CAD build for the part. Positions are in the model's coordinates, mm. A direction names the side the tool comes from. Coordinates: 2 decimals unless noted, no trailing zeros. Write each loop counter-clockwise with the first axis right and the second up, starting at its lowest first coordinate (ties: lowest second). Pieces come first, ordered by that corner, then holes. Notation, with made-up numbers: M 35,42.5 L 70,42.5 A38 ccw 70,80.5 Z; hole C 80.5,-7.5 d7. An arc over 180 degrees is marked long. Answer as CSV lines item,"result". Start each with the question number.
Autodesk Inventor part; units mm, degrees
ref_plane "YZ Plane" through (0, 0, 0) normal (1, 0, 0) x (0, 1, 0)
ref_plane "XZ Plane" through (0, 0, 0) normal (0, 1, 0) x (-1, 0, 0)
ref_plane "XY Plane" through (0, 0, 0) normal (0, 0, 1) x (1, 0, 0)
sketch "Boceto1" plane through (0, 0, 0) normal (0, 0, 1) x (1, 0, 0)
  line L0 (98.53, 89.5715) -> (-98.53, 89.5715)
  line L1 (-98.53, -89.5715) -> (98.53, 89.5715) construction
  line L2 (98.53, -89.5715) -> (-98.53, 89.5715) construction
  line L3 (3.26, -89.5715) -> (3.26, -39.0815)
  line L4 (3.26, -39.0815) -> (98.53, -39.0815)
  line L5 (98.53, 89.5715) -> (98.53, -39.0815)
  circle A0 centre (65.96, 66.7715) radius 4.5
  circle A1 centre (65.96, -18.7285) radius 4.5
  circle A2 centre (-80.61, 72.0615) radius 4.5
  circle A3 centre (-4.48, 76.5415) radius 4.5
  circle A4 centre (-80.61, -22.7985) radius 4.5
  circle A5 centre (-4.48, -40.0285) radius 4.5
  circle A6 centre (-48.45, -33.5185) radius 4.5
  circle A7 centre (-48.45, 57.2715) radius 4.5
  circle A8 centre (-48.45, 11.8765) radius 31.755
  line L6 (-83.4615, -46.0315) -> (-83.4615, -51.6915)
  line L7 (-75.3185, -51.6915) -> (-75.3185, -46.0315)
  line L8 (-83.4615, -76.9315) -> (-83.4615, -71.2715)
  line L9 (-75.3185, -71.2715) -> (-75.3185, -76.9315)
  arc A9 (-75.3185, -46.0315) -> (-83.4615, -46.0315) centre (-79.39, -46.0315) ccw
  arc A10 (-83.4615, -51.6915) -> (-75.3185, -51.6915) centre (-79.39, -51.6915) ccw
  arc A11 (-75.3185, -71.2715) -> (-83.4615, -71.2715) centre (-79.39, -71.2715) ccw
  arc A12 (-83.4615, -76.9315) -> (-75.3185, -76.9315) centre (-79.39, -76.9315) ccw
  line L10 (-19.9515, -46.0315) -> (-19.9515, -51.6915)
  line L11 (-11.8085, -51.6915) -> (-11.8085, -46.0315)
  line L12 (-19.9515, -71.2715) -> (-19.9515, -76.9315)
  line L13 (-11.8085, -71.2715) -> (-11.8085, -76.9315)
  arc A13 (-11.8085, -46.0315) -> (-19.9515, -46.0315) centre (-15.88, -46.0315) ccw
  arc A14 (-19.9515, -51.6915) -> (-11.8085, -51.6915) centre (-15.88, -51.6915) ccw
  arc A15 (-11.8085, -71.2715) -> (-19.9515, -71.2715) centre (-15.88, -71.2715) ccw
  arc A16 (-19.9515, -76.9315) -> (-11.8085, -76.9315) centre (-15.88, -76.9315) ccw
  line L14 (-98.53, 89.5715) -> (-98.53, -89.5715)
  line L15 (-98.53, -89.5715) -> (3.26, -89.5715)
  point P0 (0, 0)
  dimension "d6" = 9
  dimension "d8" = 9
  dimension "d13" = 9
  dimension "d14" = 9
  dimension "d18" = 9
  dimension "d19" = 9
  dimension "d22" = 9
  dimension "d24" = 9
  dimension "d26" = 63.51
extrude "Extrusión1" add sketch "Boceto1" along normal mid plane 0.8
fillet "Empalme1" radius 3 6 edges at (98.53, 89.5715, 0) (98.53, -39.0815, 0) (3.26, -89.5715, 0) (3.26, -39.0815, 0) (-98.53, -89.5715, 0) (-98.53, 89.5715, 0)
1) Band-saw the part on A-A, the plane x = -48.45. List the corners of the cut face in (y, z).
2) Probe L1, parallel to Y at x = -4.48, z = 0.1; L2, parallel to Y at x = -48.45, z = -0.1; L3, parallel to Y at x = 65.96, z = -0.05. List the from-to ranges inside material, lowest first. Write a range as [from, to].
3) Band-saw the part on B-B, the plane x = 65.96. List the corners of the cut face in (y, z).
4) Tool access for faces 1 (the cylindrical face through (-79.3, -55.762, -0.006)), 2 (the flat face through (-1, 1, 0.4)): list every direction of +Z, -Z, +X, -X, +Y, -Y with a clear straight run to the whole face (end or side of a thin tool).
5) Two-plate mould, pull along Y, no slides. Class faces 3 (the flat face through (-1, 1, -0.4)), 4 (the cylindrical face through (-44.158, -34.87, -0.006)), 5 (the cylindrical face through (-16, -67.2, 0)): pulls with the +Y half, pulls with the -Y half, needs draft (parallel to the pull), parting line crosses it, or undercut.
6) Band-saw the part on C-C, the plane y = -12. List the corners of the cut face in (x, z), plus the area to 3 significant figures.
7) Band-saw the part on D-D, the plane x = -28. List the corners of the cut face in (y, z).
Result sheet:
1,outline,"M -89.57,-0.4 L -38.02,-0.4 L -38.02,0.4 L -89.57,0.4 Z; M -29.02,-0.4 L -19.88,-0.4 L -19.88,0.4 L -29.02,0.4 Z; M 43.63,-0.4 L 52.77,-0.4 L 52.77,0.4 L 43.63,0.4 Z; M 61.77,-0.4 L 89.57,-0.4 L 89.57,0.4 L 61.77,0.4 Z"
2,L1,"y = [-89.57, -44.53], [-35.53, 72.04], [81.04, 89.57]"
2,L2,"y = [-89.57, -38.02], [-29.02, -19.88], [43.63, 52.77], [61.77, 89.57]"
2,L3,"y = [-39.08, -23.23], [-14.23, 62.27], [71.27, 89.57]"
3,outline,"M -39.08,-0.4 L -23.23,-0.4 L -23.23,0.4 L -39.08,0.4 Z; M -14.23,-0.4 L 62.27,-0.4 L 62.27,0.4 L -14.23,0.4 Z; M 71.27,-0.4 L 89.57,-0.4 L 89.57,0.4 L 71.27,0.4 Z"
4,face 1,"+Z, -Z"
4,face 2,"+Z, +X, -X, +Y, -Y"
5,face 3,"needs draft"
5,face 4,"undercut"
5,face 5,"undercut"
6,outline,"M -98.53,-0.4 L -69.39,-0.4 L -69.39,0.4 L -98.53,0.4 Z; M -27.51,-0.4 L 98.53,-0.4 L 98.53,0.4 L -27.51,0.4 Z"
6,area,"124 mm²"
7,outline,"M -89.57,-0.4 L -12.42,-0.4 L -12.42,0.4 L -89.57,0.4 Z; M 36.17,-0.4 L 89.57,-0.4 L 89.57,0.4 L 36.17,0.4 Z"
